```python
from build123d import *

# Parameters (mm, degrees)
ESQUISSE1_R             = 50
BOSS_EXTRU_1_DEPTH      = 3
ESQUISSE2_R             = 4
ENL_V_MAT_EXTRU_1_DEPTH = 3
ESQUISSE3_R             = 1.5
ENL_V_MAT_EXTRU_2_DEPTH = 3
R_P_T_PAR_COURBE1_COUNT = 2
ESQUISSE4_R             = 1.5
ENL_V_MAT_EXTRU_3_DEPTH = 3
R_P_T_PAR_COURBE2_COUNT = 2


with BuildPart() as part:
    # Esquisse1 → Boss.-Extru.1 (new body)
    with BuildSketch(Plane.XY):
        Circle(ESQUISSE1_R)
    extrude(amount=BOSS_EXTRU_1_DEPTH)

    # Esquisse2 → Enlèv. mat.-Extru.1 (cut)
    with BuildSketch(Plane.XY.offset(3)):
        Circle(ESQUISSE2_R)
    extrude(amount=-ENL_V_MAT_EXTRU_1_DEPTH, mode=Mode.SUBTRACT)

    # Esquisse3 → Enlèv. mat.-Extru.2 (cut)
    with BuildSketch(Plane.XY.offset(3)):
        with Locations((-44, 0)):
            Circle(ESQUISSE3_R)
    enl_v_mat_extru_2 = extrude(amount=-ENL_V_MAT_EXTRU_2_DEPTH, mode=Mode.SUBTRACT)

    # Répét. par courbe1: Enlèv. mat.-Extru.2 ×2 about axis
    r_p_t_par_courbe1_axis = Axis((0, 0, 3), (0, 0, 1))
    for i in range(1, R_P_T_PAR_COURBE1_COUNT):
        add(enl_v_mat_extru_2.rotate(r_p_t_par_courbe1_axis, i * 360 / R_P_T_PAR_COURBE1_COUNT), mode=Mode.SUBTRACT)

    # Esquisse4 → Enlèv. mat.-Extru.3 (cut)
    with BuildSketch(Plane.XY.offset(3)):
        with Locations((-33, -6)):
            Circle(ESQUISSE4_R)
    enl_v_mat_extru_3 = extrude(amount=-ENL_V_MAT_EXTRU_3_DEPTH, mode=Mode.SUBTRACT)

    # Répét. par courbe2: Enlèv. mat.-Extru.3 ×2 about axis
    r_p_t_par_courbe2_axis = Axis((0, 0, 3), (0, 0, 1))
    for i in range(1, R_P_T_PAR_COURBE2_COUNT):
        add(enl_v_mat_extru_3.rotate(r_p_t_par_courbe2_axis, i * 360 / R_P_T_PAR_COURBE2_COUNT), mode=Mode.SUBTRACT)


solid = part.part
```
Check sheet for the modelled part. Datum: model origin and axes. Units: mm. Round coordinates to 2 decimals unless told otherwise and drop trailing zeros. Order: outer loops, then holes, each group sorted by start corner. A loop starts at its lowest first (then second) coordinate and runs counter-clockwise, first axis right, second up. Notation, with made-up numbers: (-11.5, 65.25) - (11.5, 65.25) arc R26 cw to (11.5, 100.25) - close; hole circle Ø6 at (36, -34). An arc over 180 degrees is marked (long way). Answer as CSV lines item,"result". Start each with the question number.
1) Draft check along Y on faces 1 (the face through (47.69, 15.02, 1.48)), 2 (the face through (34.2, 6.9, 1.5)), 3 (the face through (-1, -10, 0)). Enter one of: +Y half, -Y half, draft (parallel to the pull), parting line (faces both ways), or undercut.
2) Section check A-A (y = 0). Record the cut outline in (x, z).
3) Scan lines: probe 1 along Y at (x, z) = (0, 0.95); probe 2 along Y at (x, z) = (-33, 1.75); probe 3 along X at (y, z) = (-12, 0.8). Record each from-to range of solid material in increasing order.
4) Section check C-C (z = 2.1). Record the cut outline in (x, y).
5) Depth check by flat-ended pin: pin 1 (1.5 mm diameter, centred on x = 19.5, z = 1.5, fed in from -Y); pin 2 (1 mm diameter, centred on x = -5, z = 2.5, fed in from -Y). Enter the tip coordinate at first touch or a pass-through.
6) Section check B-B (x = 0). Record the cut outline in (y, z).
7) Section check D-D (x = 33). Record the cut outline in (y, z).
Determined:
1,face 1,"parting line"
1,face 2,"undercut"
1,face 3,"draft"
2,outline,"(-50, 0) - (-45.5, 0) - (-45.5, 3) - (-50, 3) - close; (-42.5, 0) - (-4, 0) - (-4, 3) - (-42.5, 3) - close; (4, 0) - (42.5, 0) - (42.5, 3) - (4, 3) - close; (45.5, 0) - (50, 0) - (50, 3) - (45.5, 3) - close"
3,probe 1,"-50 to -4, 4 to 50"
3,probe 2,"-37.56 to -7.5, -4.5 to 37.56"
3,probe 3,"-48.54 to 48.54"
4,outline,"circle Ø100 at (0, 0); hole circle Ø3 at (-44, 0); hole circle Ø3 at (-33, -6); hole circle Ø8 at (0, 0); hole circle Ø3 at (33, 6); hole circle Ø3 at (44, 0)"
5,pin 1,"y = -46.35"
5,pin 2,"y = -49.8"
6,outline,"(-50, 0) - (-4, 0) - (-4, 3) - (-50, 3) - close; (4, 0) - (50, 0) - (50, 3) - (4, 3) - close"
7,outline,"(-37.56, 0) - (4.5, 0) - (4.5, 3) - (-37.56, 3) - close; (7.5, 0) - (37.56, 0) - (37.56, 3) - (7.5, 3) - close"
